The listing builds one solid part. Answer for the finished solid, in the listing's coordinates (mm). A direction names the side the tool comes from. Round coordinates to 2 decimals unless told otherwise and drop trailing zeros. Write each loop counter-clockwise with the first axis right and the second up, starting at its lowest first coordinate (ties: lowest second). Pieces come first, ordered by that corner, then holes. Notation, with made-up numbers: (-33.75, 65) - (-17.75, 65) arc R29 cw to (-17.75, 100) - close; hole circle Ø6 at (88.5, -38). An arc over 180 degrees is marked (long way). Answer in a Markdown table with one row per item.
from build123d import *

# Parameters (mm, degrees)
EXTRUDE_1_DEPTH     = 6.1
EXTRUDE_2_DEPTH     = 4.3
SKETCH_3_R          = 2.5
EXTRUDE_3_DEPTH     = 2.6
SWEEP_START         = -2
SWEEP_1_DEPTH       = 4
CUT_EXTRUDE_1_DEPTH = 3


# Read off the part's stored shape, not the designer's step: По траектории1
with BuildPart() as part:
    # Эскиз1 → Бобышка-Вытянуть1 (new, symmetric)
    with BuildSketch(Plane(origin=(0, 0, 0), x_dir=(0, 0, -1), z_dir=(1, 0, 0))):
        Polygon((0, 0), (22.3, 0), (22.3, 15.8), (27, 15.8), (27, 18.1), (22.3, 18.1), (22.3, 22.2), (0, 22.2), (0, 18.1), (-4.7, 18.1), (-4.7, 15.8), (0, 15.8), align=None)
    extrude(amount=EXTRUDE_1_DEPTH, both=True)

    # Эскиз2 → Бобышка-Вытянуть2 (add)
    with BuildSketch(Plane(origin=(0, 22.2, 0), x_dir=(1, 0, 0), z_dir=(0, 1, 0))):
        with BuildLine():
            Line((-2.75, 12.2), (-2.75, 11.54495179))
            ThreePointArc((-2.75, 11.54495179), (0, 0), (2.75, 11.54495179))
            Line((2.75, 11.54495179), (2.75, 12.2))
            ThreePointArc((2.75, 12.2), (0, 14.95), (-2.75, 12.2))
        make_face()
    extrude(amount=EXTRUDE_2_DEPTH)

    # Эскиз3 → Бобышка-Вытянуть3 (add)
    with BuildSketch(Plane(origin=(0, 26.5, 0), x_dir=(1, 0, 0), z_dir=(0, 1, 0))):
        with Locations(Location((0, 6.1, 0), (0, 0, 270))):
            Circle(SKETCH_3_R)
    extrude(amount=EXTRUDE_3_DEPTH)

    # По траектории1 outline → По траектории1 (add)
    with BuildSketch(Plane.YZ.offset(SWEEP_START)):
        with BuildLine():
            Line((5, 0), (7.5, 0))
            add(Edge.make_bspline(
                [(7.5, 0), (7.55466995, 0.932768751), (7.567397074, 2.054373731), (7.427446861, 3.871339503), (7.144525851, 5.668082774), (6.567191568, 7.327579523), (5.845700953, 8.750774075), (5.129629815, 9.89551827), (4.584016429, 10.917508592), (4.409004277, 11.592638933), (4.374327462, 11.966191087), (4.40728466, 12.331644555), (4.518227027, 12.728854054), (4.738611449, 13.18957707), (4.985731728, 13.5588281), (5.139543938, 13.750446366)],
                knots=[0, 0, 0, 0, 0.166666667, 0.203301869, 0.333333333, 0.5, 0.519938297, 0.625, 0.75, 0.791666667, 0.833333333, 0.875, 0.916666667, 0.958333333, 1, 1, 1, 1], degree=3))
            Line((5.139543938, 13.750446366), (3.063253187, 15.142932171))
            add(Edge.make_bspline(
                [(5, 0), (5.057281604, 0.840170125), (5.073194453, 1.848822262), (4.963561919, 3.425294528), (4.739313637, 4.934487741), (4.312374062, 6.230912608), (3.740083573, 7.399180935), (3.13051994, 8.398930623), (2.368002426, 9.70405156), (1.994241871, 10.907667376), (1.874475502, 11.699413606), (1.900467078, 12.546155788), (2.099949953, 13.416272622), (2.478763958, 14.286542274), (2.848255397, 14.852807038), (3.063253187, 15.142932171)],
                knots=[0, 0, 0, 0, 0.166666667, 0.203301869, 0.333333333, 0.5, 0.519938297, 0.625, 0.75, 0.791666667, 0.833333333, 0.875, 0.916666667, 0.958333333, 1, 1, 1, 1], degree=3))
        make_face()
    extrude(amount=SWEEP_1_DEPTH)

    # Эскиз6 → Вырез-Вытянуть1 (cut)
    with BuildSketch(Plane(origin=(0, 18.1, 0), x_dir=(1, 0, 0), z_dir=(0, 1, 0))):
        with BuildLine():
            Line((-0.5, 27), (-0.5, 25.795643924))
            ThreePointArc((-0.5, 25.795643924), (0, 23.4), (0.5, 25.795643924))
            Line((0.5, 25.795643924), (0.5, 27))
            Line((0.5, 27), (0, 27))
            Line((0, 27), (-0.5, 27))
        make_face()
        with BuildLine():
            Line((0.5, -4.7), (0.5, -3.495643924))
            ThreePointArc((0.5, -3.495643924), (0, -1.1), (-0.5, -3.495643924))
            Line((-0.5, -3.495643924), (-0.5, -4.7))
            Line((-0.5, -4.7), (0, -4.7))
            Line((0, -4.7), (0.5, -4.7))
        make_face()
    extrude(amount=-CUT_EXTRUDE_1_DEPTH, mode=Mode.SUBTRACT)


solid = part.part
(1) Section B-B (y = 16.75) is taken. Give the vertices of the cut face in (x, z).
Checked values:
| item | result |
|---|---|
| outline | (-6.1, -27) - (-0.5, -27) - (-0.5, -25.8) arc R1.25 cw (long way) to (0.5, -25.8) - (0.5, -27) - (6.1, -27) - (6.1, 4.7) - (0.5, 4.7) - (0.5, 3.5) arc R1.25 cw (long way) to (-0.5, 3.5) - (-0.5, 4.7) - (-6.1, 4.7) - close |
(2) Find the intervals of material crossed by line 1 (X direction, y = 16.8, z = -24.65); line 2 (Z direction, x = 0, y = 16.7); line 3 (Y direction, x = -0.75, z = -14), in increasing order.
Checked values:
| item | result |
|---|---|
| line 1 | x = -6.1 to -1.25, 1.25 to 6.1 |
| line 2 | z = -23.4 to 1.1 |
| line 3 | y = 0 to 26.5 |
(3) For a pull along X with two mould halves and no side action, classify faces 1 (the flat face through (-0.028, 4.116, 14.437)), 2 (the flat face through (2, 5, 8)), 3 (the cylindrical face through (0, 24, 0)), 4 (the flat face through (0.5, 17, 4)) as pulls with the +X half, pulls with the -X half, needs draft (parallel to the pull), parting line crosses it, or undercut.
Checked values:
| item | result |
|---|---|
| face 1 | needs draft |
| face 2 | pulls with the +X half |
| face 3 | parting line crosses it |
| face 4 | undercut |
(4) Flat-ended cylindrical pins translate along their axes: pin 1 (0.5 mm diameter, centred on y = 24, z = -12, fed in from -X); pin 2 (3 mm diameter, centred on x = 0.5, y = 12.5, fed in from -Z); pin 3 (0.7 mm diameter, centred on x = -2, y = 16.5, fed in from +Z). Find the tip coordinate at first contact, or state that the pin passes through.
Checked values:
| item | result |
|---|---|
| pin 1 | stops at x = -2.75 |
| pin 2 | stops at z = -22.3 |
| pin 3 | stops at z = 4.7 |
(5) Section A-A (z = -24.65) is taken. Give the vertices of the cut face in (x, y).
Checked values:
| item | result |
|---|---|
| outline | (-6.1, 15.8) - (-1.25, 15.8) - (-1.25, 18.1) - (-6.1, 18.1) - close; (1.25, 15.8) - (6.1, 15.8) - (6.1, 18.1) - (1.25, 18.1) - close |
(6) Section C-C (x = -5) is taken. Give the vertices of the cut face in (y, z), and give its area (3 significant figures).
Checked values:
| item | result |
|---|---|
| outline | (0, -22.3) - (15.8, -22.3) - (15.8, -27) - (18.1, -27) - (18.1, -22.3) - (22.2, -22.3) - (22.2, -9.59) - (26.5, -9.59) - (26.5, -2.61) - (22.2, -2.61) - (22.2, 0) - (18.1, 0) - (18.1, 4.7) - (15.8, 4.7) - (15.8, 0) - (0, 0) - close |
| area | 547 mm2 |
(7) For faces 5 (the flat face through (3, 17, 4.7)), 6 (the flat face through (5, 22.2, -1)), 7 (the flat face through (0.5, 17, -26)), 8 (the flat face through (0, 8, -22.3)), 9 (the flat face through (1.4, 15.8, 2.4)), determine the directions among +Z, -Z, +X, -X, +Y, -Y from which every point of the face is accessible in a straight line to the end or side of a thin tool.
Checked values:
| item | result |
|---|---|
| face 5 | +Z, +X, -X, +Y |
| face 6 | +Z, +X, +Y |
| face 7 | -Z, +Y, -Y |
| face 8 | -Z, +X, -X, -Y |
| face 9 | +Z, +X, -X |
(8) Section D-D (z = -1) is taken. Give the vertices of the cut face in (x, y).
Checked values:
| item | result |
|---|---|
| outline | (-6.1, 0) - (6.1, 0) - (6.1, 22.2) - (3.35, 22.2) - (3.35, 26.5) - (-3.35, 26.5) - (-3.35, 22.2) - (-6.1, 22.2) - close |
